```python
from build123d import *

# Parameters (mm, degrees)
IZIM1_W                     = 76.2
IZIM1_H                     = 19.05
IZIM1_R                     = 2.38
Y_KSEKLIK_EKSTR_ZYON1_DEPTH = 6.35


with BuildPart() as part:
    # Çizim1 → Yükseklik-Ekstrüzyon1 (new body)
    with BuildSketch(Plane(origin=(0, 0, 0), x_dir=(1, 0, 0), z_dir=(0, 1, 0))):
        with Locations((-3.015107914, 6.715467626)):
            Rectangle(IZIM1_W, IZIM1_H)
        with Locations(Location((-31.765107914, 6.715467626, 0), (0, 0, 270))):
            Circle(IZIM1_R, mode=Mode.SUBTRACT)
        with BuildLine():
            Line((30.324892086, 10.182112257), (30.324892086, 3.248822995))
            ThreePointArc((30.324892086, 3.248822995), (19.349892086, 6.715467626), (30.324892086, 10.182112257))
        make_face(mode=Mode.SUBTRACT)
    extrude(amount=Y_KSEKLIK_EKSTR_ZYON1_DEPTH)


solid = part.part
```
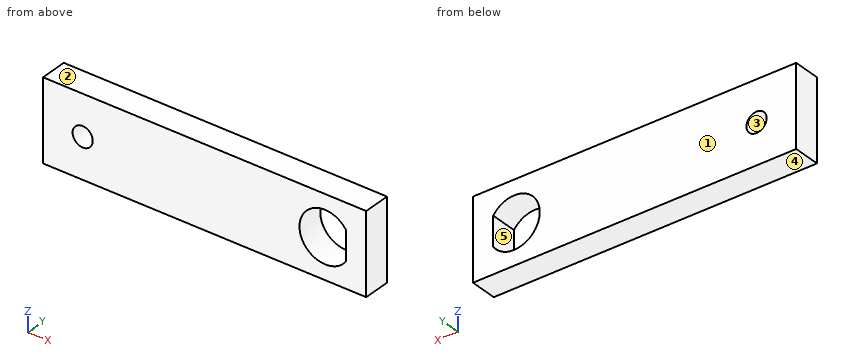
Model file for the job. Use its own axes, mm. Face numbers are marked on the shaded views. A direction names the side the tool comes from. Round coordinates to 2 decimals unless told otherwise and drop trailing zeros. Write each loop counter-clockwise with the first axis right and the second up, starting at its lowest first coordinate (ties: lowest second). Pieces come first, ordered by that corner, then holes. Notation, with made-up numbers: (79.5, 51.25) - (115.5, 51.25) arc R11 ccw to (115.5, 65.25) - close; hole circle Ø6 at (59, 15.5). An arc over 180 degrees is marked (long way). One line per item, written item: value.
(1) Wall check: probe 1 along X at (y, z) = (1, -8); probe 2 along X at (y, z) = (3.5, -7); probe 3 along Z at (x, y) = (20, 4.5). Give the ranges that are in metal, low to high.
Values follow:
probe 1: x = -41.12 to -33.77, -29.76 to 19.49, 30.32 to 35.08
probe 2: x = -41.12 to -34.13, -29.4 to 19.36, 30.32 to 35.08
probe 3: z = -16.24 to -9.44, -3.99 to 2.81
(2) Cut at A-A, the plane z = -1.75. Give the cut face in (x, y).
Values follow:
outline: (-41.12, 0) - (21.95, 0) - (21.95, 6.35) - (-41.12, 6.35) - close; (28.81, 0) - (35.08, 0) - (35.08, 6.35) - (28.81, 6.35) - close
(3) Cut at B-B, the plane z = -7. Give the cut face in (x, y), plus the area to 3 significant figures.
Values follow:
outline: (-41.12, 0) - (-34.13, 0) - (-34.13, 6.35) - (-41.12, 6.35) - close; (-29.4, 0) - (19.36, 0) - (19.36, 6.35) - (-29.4, 6.35) - close; (30.32, 0) - (35.08, 0) - (35.08, 6.35) - (30.32, 6.35) - close
area: 384 mm²
(4) Two-plate mould, pull along Z, no slides. Class the marked faces 1, 2 and 3: pulls with the +Z half, pulls with the -Z half, needs draft (parallel to the pull), parting line crosses it, or undercut.
Values follow:
face 1: needs draft
face 2: pulls with the +Z half
face 3: undercut
(5) 3-axis set-ups, long thin cutter, end or side, ignore diameter. For the marked faces 4 and 5: which of +Z, -Z, +X, -X, +Y, -Y reach the whole face in a straight line?
Values follow:
face 4: -Z, +X, -X, +Y, -Y
face 5: +Y, -Y
(6) Cut at D-D, the plane y = 4. Give the cut face in (x, z) (3 decimals).
Values follow:
outline: (-41.115, -16.24) - (35.085, -16.24) - (35.085, 2.81) - (-41.115, 2.81) - close; hole circle Ø4.76 at (-31.765, -6.715); hole (30.325, -10.182) - (30.325, -3.249) arc R6.035 ccw (long way) to start
(7) Cut at C-C, the plane x = 25.5. Give the cut face in (y, z).
Values follow:
outline: (0, -16.24) - (6.35, -16.24) - (6.35, -12.75) - (0, -12.75) - close; (0, -0.68) - (6.35, -0.68) - (6.35, 2.81) - (0, 2.81) - close
